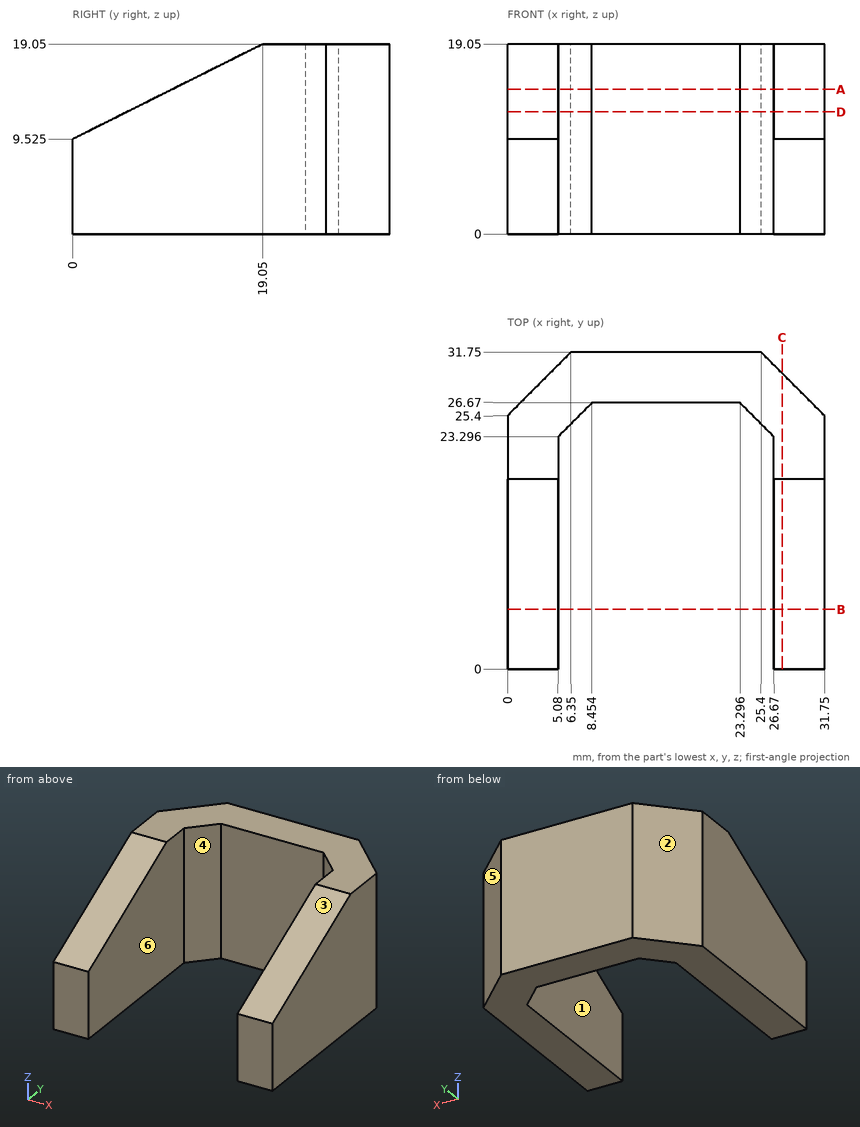
Drawing for the job (mm, zero at the part's lowest x, y, z). A direction names the side the tool comes from. Give positions to 0.01 mm unless a question says otherwise; leave off trailing zeros. Order: outer loops, then holes, each group sorted by start corner. A loop starts at its lowest first (then second) coordinate and runs counter-clockwise, first axis right, second up. Notation, with made-up numbers: (-12.75, 40.5) - (38.25, 40.5) arc R14 cw to (38.25, 57.5) - close; hole circle Ø7 at (14.5, -21). An arc over 180 degrees is marked (long way). Write item = value, one per line. Start each with the question number.
1. Cut at A-A, the plane z = 14.5. List the corners of the cut face in (x, y).
2. Drop a flat-ended pin along its axis: P1, Ø10, axis at x = 5.5, y = 23.5, coming from the -Z side. Give the stop position or say it passes through.
3. Cut at D-D, the plane z = 12.25. List the corners of the cut face in (x, y).
4. Cut at B-B, the plane y = 6. List the corners of the cut face in (x, z) (3 decimals).
5. Two-plate mould, pull along X, no slides. Class the marked faces 3, 4, 5 and 6: pulls with the +X half, pulls with the -X half, needs draft (parallel to the pull), parting line crosses it, or undercut.
6. Which spindle directions (+Z, -Z, +X, -X, +Y, -Y) get a long thin tool onto all of the face, cutting with end or side? Do the marked faces 1 and 2. Say none if no direction does.
7. Probe line 1 along X through (y, z) = (14.5, 12.5); line 2 along Y through (x, z) = (13.5, 8.75); line 3 along Y through (x, z) = (6, 9) (1 decimal). List the from-to ranges inside material, lowest first.
8. Cut at C-C, the plane x = 27.5. List the corners of the cut face in (y, z) (3 decimals), and give its area (3 significant figures).
Taken from the geometry:
q1.outline = (0, 9.95) - (5.08, 9.95) - (5.08, 23.3) - (8.45, 26.67) - (23.3, 26.67) - (26.67, 23.3) - (26.67, 9.95) - (31.75, 9.95) - (31.75, 25.4) - (25.4, 31.75) - (6.35, 31.75) - (0, 25.4) - close
q2.P1 = 0
q3.outline = (0, 5.45) - (5.08, 5.45) - (5.08, 23.3) - (8.45, 26.67) - (23.3, 26.67) - (26.67, 23.3) - (26.67, 5.45) - (31.75, 5.45) - (31.75, 25.4) - (25.4, 31.75) - (6.35, 31.75) - (0, 25.4) - close
q4.outline = (0, 0) - (5.08, 0) - (5.08, 12.525) - (0, 12.525) - close; (26.67, 0) - (31.75, 0) - (31.75, 12.525) - (26.67, 12.525) - close
q5.face_3 = needs draft
q5.face_4 = undercut
q5.face_5 = pulls with the +X half
q5.face_6 = undercut
q6.face_1 = +Z, -Z, -Y
q6.face_2 = +Z, -Z, -X, +Y
q7.line_1 = 0 to 5.08, 26.67 to 31.75
q7.line_2 = 26.67 to 31.75
q7.line_3 = 24.2 to 31.4
q8.outline = (0, 0) - (29.65, 0) - (29.65, 19.05) - (19.05, 19.05) - (0, 9.525) - close
q8.area = 474 mm²
